from build123d import *

# Parameters (mm, degrees)
F0_R     = 17.9
F0_R_2   = 16.5
F1_DEPTH = 25
F3_DEPTH = 2
F4_W     = 2
F4_H     = 3
F4_H_2   = 2
F5_DEPTH = 1
F6_R     = 0.99999
F7_R     = 4
F8_SIZE2 = 0.1099571106
F8_SIZE  = 18


# Not quite as in the source:
# - a fillet or chamfer is up to 0.001 mm smaller than in the source, because OpenCascade refuses the exact size


with BuildPart() as f1:
    # F0 (on Top) → F1 (new body)
    with BuildSketch(Plane.XY):
        Circle(F0_R)
        Circle(F0_R_2, mode=Mode.SUBTRACT)
    extrude(amount=-F1_DEPTH)

    # F0 (on Top) → F3 (join)
    with BuildSketch(Plane.XY):
        Circle(F0_R_2)
    extrude(amount=-F3_DEPTH)

    # F4 (on face) → F5 (join, symmetric)
    with BuildSketch(Plane.XZ):
        Polygon((6, 4), (6, 0), (8, 0), (8, 6), (6, 6), align=None)
        with Locations((-7, 2.5)):
            Rectangle(F4_W, F4_H)
        with Locations((-7, 5)):
            Rectangle(F4_W, F4_H_2)
        Polygon((-4, 4), (6, 4), (6, 6), (-6, 6), (-6, 4), align=None)
    extrude(amount=F5_DEPTH, both=True)

    # F6 (radius 1 in the source; OpenCascade refuses exactly that, so slightly less here)
    f6_edges = [f1.edges().sort_by_distance(p)[0] for p in [
        (8, 0, 0),
        (7, -1, 0),
        (7, 1, 0),
        (6, 0, 4),
        (-6, 0, 4),
        (8, 0, 6),
        (-8, 0, 6),
        (6, 0, 0),
        (-8, 0, 1),
        (-6, 0, 1),
        (0, -1, 6),
        (0, 1, 6),
    ]]
    fillet(f6_edges, radius=F6_R)

    # F7
    f7_edges = [f1.edges().sort_by_distance(p)[0] for p in [
        (-17.9, 0, 0),
        (-16.5, 0, -2),
    ]]
    fillet(f7_edges, radius=F7_R)

    # F8
    f8_edges = [f1.edges().sort_by_distance(p)[0] for p in [
        (-16.5, 0, -25),
    ]]
    f8_side = f1.faces().sort_by_distance((-16.5, 0, -15.5))[0]
    chamfer(f8_edges, length=F8_SIZE, length2=F8_SIZE2, reference=f8_side)


solid = f1.part
Read the model definition and answer for the solid it produces. Units are mm, in the model's axes. A direction names the side the tool comes from. Coordinates: 2 decimals unless noted, no trailing zeros. Write each loop counter-clockwise with the first axis right and the second up, starting at its lowest first coordinate (ties: lowest second). Pieces come first, ordered by that corner, then holes. Notation, with made-up numbers: (89.25, 54.25) -> (138.25, 54.25) arc R29 ccw to (138.25, 84.25) -> close; hole circle Ø7 at (85.5, 22.5). An arc over 180 degrees is marked (long way). Return JSON: item names as keys, results as strings.
(1) Which of the six approach directions +Z, -Z, +X, -X, +Y, -Y give full straight-line access (tool end or side, diameter ignored) to faces 4 (the flat face through (-8, 0, 4)), 5 (the flat face through (0, 0, 4)), 6 (the flat face through (8, 0, 3))?
Answers below:
{"face 4": "+Z, -X, +Y, -Y", "face 5": "+Y, -Y", "face 6": "+Z, +X, +Y, -Y"}
(2) Consider line 1 along Y through (x, z) = (0, -6.45); line 2 along Z through (x, y) = (11, 3.5); line 3 along X through (y, z) = (8, -7.5). Determine where each line is inside the solid, lowest interval first. Write a range as from..to.
Answers below:
{"line 1": "-17.9..-16.5, 16.5..17.9", "line 2": "-2..0", "line 3": "-16.01..-14.43, 14.43..16.01"}
(3) The part is cut by section B-B on z = -13. Give the vertices of the cut face in (x, y).
Answers below:
{"outline": "circle Ø35.8 at (0, 0); hole circle Ø33.07 at (0, 0)"}
(4) For a pull along X with two mould halves and no side action, classify faces 1 (the cylindrical face through (5.715, 0.014, 3.699)), 2 (the flat face through (-0.1, -1, 4.4)), 3 (the cylindrical face through (8.4, 0, 0.2)) as pulls with the +X half, pulls with the -X half, needs draft (parallel to the pull), parting line crosses it, or undercut.
Answers below:
{"face 1": "undercut", "face 2": "needs draft", "face 3": "pulls with the +X half"}
(5) The part is cut by section A-A on z = -9. Give the vertices of the cut face in (x, y), then the cut area to 3 significant figures.
Answers below:
{"outline": "circle Ø35.8 at (0, 0); hole circle Ø33.02 at (0, 0)", "area": "150 mm^2"}
(6) Each of these flat-tipped pins is pushed along its axis until it touches: P1, Ø1.1, axis at y = -0.5, z = 2.5, coming from the +X side; P2, Ø4, axis at x = 13.5, z = -16.5, coming from the -Y side; P3, Ø2, axis at x = 9.5, z = -2.5, coming from the +Y side. Where does it stop, or does it pass through?
Answers below:
{"P1": "x = 8", "P2": "y = -13.72", "P3": "y = 15.54"}
